```python
from build123d import *

# Parameters (mm, degrees)
F0_W      = 38.1
F0_H      = 38.1
F1_DEPTH  = 38.1
F6_DEPTH  = 38.1
F8_DEPTH  = 38.1
F9_W      = 25.4
F9_H      = 7.62
F10_DEPTH = 38.1


with BuildPart() as f1:
    # F0 (on Front) → F1 (new body)
    with BuildSketch(Plane.XZ):
        with Locations((19.05, 19.05)):
            Rectangle(F0_W, F0_H)
    extrude(amount=F1_DEPTH)

    # F5 (on offset) → F6 (cut)
    with BuildSketch(Plane.YZ.offset(38.1)):
        Polygon((-11.43, 15.875), (-6.35, 38.1), (-31.75, 38.1), (-26.67, 15.875), (-21.59, 28.575), (-16.51, 28.575), align=None)
        Polygon((-31.75, 0), (-38.1, 38.1), (-38.1, 0), align=None)
        Polygon((-6.35, 0), (0, 0), (0, 38.1), align=None)
        Polygon((-25.4, 0), (-12.7, 0), (-19.05, 15.875), align=None)
    extrude(amount=-F6_DEPTH, mode=Mode.SUBTRACT)

    # F7 (on offset) → F8 (cut)
    with BuildSketch(Plane.XZ.offset(38.1)):
        Polygon((25.4, 38.1), (12.7, 38.1), (19.05, 24.545955), align=None)
        Polygon((11.43, 22.225), (6.35, 0), (31.75, 0), (26.67, 22.225), (21.59, 9.525), (16.51, 9.525), align=None)
        Polygon((31.75, 38.1), (38.1, 0), (38.1, 38.1), align=None)
        Polygon((0, 38.1), (0, 0), (6.35, 38.1), align=None)
    extrude(amount=-F8_DEPTH, mode=Mode.SUBTRACT)

    # F9 (on offset) → F10 (cut)
    with BuildSketch(Plane.XY.offset(38.1)):
        with Locations((25.4, -11.43)):
            Rectangle(F9_W, F9_H)
        with Locations((12.7, -26.67)):
            Rectangle(F9_W, F9_H)
    extrude(amount=-F10_DEPTH, mode=Mode.SUBTRACT)


solid = f1.part
```
Geometry check sheet. Reference: the model listing, model coordinates, mm. A direction names the side the tool comes from. Coordinates: 2 decimals unless noted, no trailing zeros. Write each loop counter-clockwise with the first axis right and the second up, starting at its lowest first coordinate (ties: lowest second). Pieces come first, ordered by that corner, then holes. Notation, with made-up numbers: M 75.5,73.5 L 92.5,73.5 A13 ccw 92.5,78.5 Z; hole C 70.25,21 d8. An arc over 180 degrees is marked long. Use one line per item in the form item = value. Start each with the question number.
1) Release check for a two-part mould opening along X. For faces 4 (the flat face through (3.836, -33.497, 23.017)), 5 (the flat face through (24.166, -5.72, 15.964)), 6 (the flat face through (9.063, -8.926, 26.832)) record: pulls with the +X half, pulls with the -X half, needs draft (parallel to the pull), parting line crosses it, or undercut.
2) Thickness scan on probe 1 along Y at (x, z) = (17.5, 20); probe 2 along Y at (x, z) = (19, 19.5); probe 3 along X at (y, z) = (-4, 21). Record the ranges inside material, lowest first. Write a range as from..to.
3) Section check A-A on z = 5. Enter the section's corners in (x, y), and give its area (3 significant figures).
4) Go/stop test with flat-tipped pins: pin 1 Ø1.5 at (x, y) = (8.5, -19) entering from +Z (3 decimals); pin 2 Ø0.6 at (x, y) = (18, -15.5) entering from -Z (3 decimals); pin 3 Ø2.5 at (y, z) = (-29, 23.5) entering from -X. Record where each tip stops, or that it passes through.
5) Section check B-B on x = 18. State how many separate pieces and enclosed holes the cut face has, and give its area (3 significant figures).
6) Set-up check for faces 1 (the flat face through (19, -6, 9.525)), 2 (the flat face through (15.83, -3.86, 31.42)), 3 (the flat face through (25.4, -30, 23)): record each of +Z, -Z, +X, -X, +Y, -Y from which the full face is reachable in a straight line by a thin tool's end or side.
7) Section check D-D on z = 29.5. Enter the section's corners in (x, y), and give its area (3 significant figures).
Responses:
q1.face_4 = pulls with the -X half
q1.face_5 = undercut
q1.face_6 = needs draft
q2.probe_1 = -35.08..-30.48, -22.86..-15.24, -7.62..-3.02
q2.probe_2 = -35..-30.48, -22.86..-15.24, -7.62..-3.1
q2.probe_3 = 3.5..11.15, 11.92..26.18, 26.95..34.6
q3.outline = M 0.83,-32.58 L 7.49,-32.58 L 7.49,-30.48 L 0.83,-30.48 Z; M 0.83,-14.7 L 7.49,-14.7 L 7.49,-5.52 L 0.83,-5.52 Z; M 30.61,-32.58 L 37.27,-32.58 L 37.27,-23.4 L 30.61,-23.4 Z; M 30.61,-7.62 L 37.27,-7.62 L 37.27,-5.52 L 30.61,-5.52 Z
q3.area = 150 mm2
q4.pin_1 = 28.575
q4.pin_2 = 9.525
q4.pin_3 = 25.4
q5.separate_pieces = 3
q5.enclosed_holes = 0
q5.area = 263 mm2
q6.face_1 = -Z, +Y, -Y
q6.face_2 = +Z, +Y, -Y
q6.face_3 = +Z, -Z, -X
q7.outline = M 4.92,-36.67 L 16.73,-36.67 L 16.73,-30.48 L 4.92,-30.48 Z; M 4.92,-8.32 L 12.7,-8.32 L 12.7,-7.62 L 16.73,-7.62 L 16.73,-1.43 L 4.92,-1.43 Z; M 21.37,-36.67 L 33.18,-36.67 L 33.18,-29.78 L 25.4,-29.78 L 25.4,-30.48 L 21.37,-30.48 Z; M 21.37,-7.62 L 33.18,-7.62 L 33.18,-1.43 L 21.37,-1.43 Z
q7.area = 303 mm2
